Check sheet for the modelled part. Datum: model origin and axes. Units: mm. Give positions to 0.01 mm unless a question says otherwise; leave off trailing zeros. Order: outer loops, then holes, each group sorted by start corner. A loop starts at its lowest first (then second) coordinate and runs counter-clockwise, first axis right, second up.
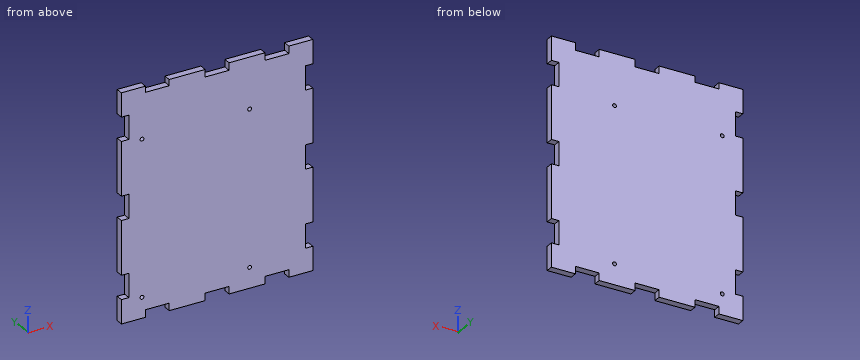
Autodesk Inventor part; units mm, degrees
ref_plane "YZ Plane" through (0, 0, 0) normal (1, 0, 0) x (0, 1, 0)
ref_plane "XZ Plane" through (0, 0, 0) normal (0, 1, 0) x (-1, 0, 0)
ref_plane "XY Plane" through (0, 0, 0) normal (0, 0, 1) x (1, 0, 0)
sketch "Fundo" plane through (0, 0, 0) normal (0, 1, 0) x (-1, 0, 0)
  line L0 (0, 0) -> (-80, 0)
  line L1 (-80, 0) -> (-80, -95)
  line L2 (-80, -95) -> (0, -95)
  line L3 (0, -95) -> (0, 0)
  dimension "d0" = 80
  dimension "d1" = 95
extrude "Extrusão1" add sketch "Fundo" along normal blind 3
sketch "Esboço3" plane through (0, 3, 0) normal (0, 1, 0) x (1, 0, 0)
  line L0 (10, -0.55) -> (20, -0.55)
  line L1 (20, -0.55) -> (20, 2.55)
  line L2 (20, 2.55) -> (10, 2.55)
  line L3 (10, 2.55) -> (10, -0.55)
  line L4 (0, 0) -> (80, 0)
  line L5 (70, 0) -> (60, 0)
  line L6 (60, 0) -> (60, 3.1)
  line L7 (60, 3.1) -> (70, 3.1)
  line L8 (70, 3.1) -> (70, 0)
  line L9 (35, 0) -> (45, 0)
  line L10 (45, 0) -> (45, 3.1)
  line L11 (45, 3.1) -> (35, 3.1)
  line L12 (35, 3.1) -> (35, 0)
  line L13 (80, 95) -> (0, 95)
  line L14 (10, 95) -> (20, 95)
  line L15 (20, 95) -> (20, 91.9)
  line L16 (20, 91.9) -> (10, 91.9)
  line L17 (10, 91.9) -> (10, 95)
  line L18 (35, 95) -> (45, 95)
  line L19 (45, 95) -> (45, 91.9)
  line L20 (45, 91.9) -> (35, 91.9)
  line L21 (35, 91.9) -> (35, 95)
  line L22 (60, 95) -> (70, 95)
  line L23 (70, 95) -> (70, 91.9)
  line L24 (70, 91.9) -> (60, 91.9)
  line L25 (60, 91.9) -> (60, 95)
  line L26 (80, 0) -> (80, 95)
  line L27 (0, 95) -> (0, 0)
  point P0 (10, 1)
  point P1 (60, 1.55)
  point P2 (20, 1)
  point P3 (35, 1.55)
  point P4 (10, 93.45)
  point P5 (70, 93.45)
  point P6 (60, 93.45)
  point P7 (45, 93.45)
  point P8 (45, 1.55)
  point P9 (35, 93.45)
  point P10 (20, 93.45)
  point P11 (20, 95)
  point P12 (45, 0)
  point P13 (60, 0)
  point P14 (70, 1.55)
  dimension "d4" = 10
  dimension "d5" = 3.1
  dimension "d7" = 10
  dimension "d8" = 3.1
  dimension "d10" = 10
  dimension "d11" = 3.1
  dimension "d18" = 10
  dimension "d19" = 3.1
  dimension "d20" = 10
  dimension "d21" = 3.1
  dimension "d22" = 10
  dimension "d23" = 3.1
  dimension "d30" = 10
  dimension "d113" = 10
  dimension "d114" = 10
  dimension "d115" = 15
  dimension "d116" = 15
  dimension "d117" = 40
  dimension "d118" = 15
  dimension "d119" = 15
  dimension "d120" = 10
extrude "Extrusão2" cut sketch "Esboço3" against normal blind 10 contours L3 L4 L1 L0 | L3 L2 L1 L4 | L12 L11 L10 L4 | L13 L15 L16 L17 | L6 L7 L8 L4 | L13 L19 L20 L21 | L13 L23 L24 L25
sketch "Esboço4" plane through (0, 3, 0) normal (0, 1, 0) x (1, 0, 0)
  line L0 (0, 95) -> (0, 0)
  line L1 (0, 10) -> (3.1, 10)
  line L2 (3.1, 10) -> (3.1, 20)
  line L3 (3.1, 20) -> (0, 20)
  line L4 (0, 20) -> (0, 10)
  line L5 (0, 85) -> (3.1, 85)
  line L6 (3.1, 85) -> (3.1, 75)
  line L7 (3.1, 75) -> (0, 75)
  line L8 (0, 75) -> (0, 85)
  line L9 (0, 42.5) -> (3.1, 42.5)
  line L10 (3.1, 42.5) -> (3.1, 52.5)
  line L11 (3.1, 52.5) -> (0, 52.5)
  line L12 (0, 52.5) -> (0, 42.5)
  line L13 (10, 95) -> (0, 95)
  line L14 (80, 0) -> (80, 95)
  line L15 (80, 10) -> (76.9, 10)
  line L16 (76.9, 10) -> (76.9, 20)
  line L17 (76.9, 20) -> (80, 20)
  line L18 (80, 20) -> (80, 10)
  line L19 (80, 42.5) -> (76.9, 42.5)
  line L20 (76.9, 42.5) -> (76.9, 52.5)
  line L21 (76.9, 52.5) -> (80, 52.5)
  line L22 (80, 52.5) -> (80, 42.5)
  line L23 (80, 75) -> (76.9, 75)
  line L24 (76.9, 75) -> (76.9, 85)
  line L25 (76.9, 85) -> (80, 85)
  line L26 (80, 85) -> (80, 75)
  line L27 (70, 0) -> (80, 0)
  line L28 (80, 95) -> (70, 95)
  point P0 (1.55, 10)
  point P1 (1.55, 85)
  point P2 (1.55, 75)
  point P3 (1.55, 52.5)
  point P4 (1.55, 20)
  point P5 (78.45, 10)
  point P6 (78.45, 85)
  point P7 (78.45, 52.5)
  point P8 (78.45, 75)
  point P9 (80, 85)
  point P10 (0, 75)
  point P11 (0, 52.5)
  point P12 (0, 20)
  point P13 (78.45, 42.5)
  point P14 (78.45, 20)
  dimension "d44" = 3.1
  dimension "d45" = 10
  dimension "d46" = 10
  dimension "d47" = 3.1
  dimension "d48" = 10
  dimension "d49" = 10
  dimension "d50" = 10
  dimension "d51" = 22.5
  dimension "d53" = 3.1
  dimension "d54" = 10
  dimension "d55" = 3.1
  dimension "d56" = 10
  dimension "d57" = 3.1
  dimension "d58" = 10
  dimension "d59" = 10
  dimension "d60" = 10
  dimension "d61" = 22.5
  dimension "d64" = 22.5
  dimension "d130" = 55
extrude "Extrusão3" cut sketch "Esboço4" against normal blind 10
sketch "Esboço6" plane through (0, 3, 0) normal (0, 1, 0) x (1, 0, 0)
  line L0 (8.6, 86.4) -> (53.6, 86.4)
  line L1 (53.6, 86.4) -> (53.6, 21.4)
  line L2 (53.6, 21.4) -> (8.6, 21.4)
  line L3 (8.6, 21.4) -> (8.6, 86.4)
  line L4 (3.1, 85) -> (3.1, 75)
  line L5 (20, 91.9) -> (10, 91.9)
  circle A0 centre (53.6, 86.4) radius 0.8
  circle A1 centre (53.6, 21.4) radius 0.8
  circle A2 centre (8.6, 21.4) radius 0.8
  circle A3 centre (8.6, 86.4) radius 0.8
  point P0 (0, 0)
  point P1 (3.1, 80)
  point P2 (15, 91.9)
  dimension "d134" = 65
  dimension "d135" = 45
  dimension "d136" = 5.5
  dimension "d137" = 5.5
  dimension "d138" = 1.6
  dimension "d139" = 1.6
  dimension "d140" = 1.6
  dimension "d141" = 1.6
extrude "Extrusão4" cut sketch "Esboço6" against normal blind 10 contours L3 A3 L0 | L0 A3 L3 | A0 L1 L0 | L0 L1 A0 | A2 L2 L3 | L3 L2 A2 | A1 L2 L1 | L1 L2 A1
properties part number "Fundo"
(1) Gauge pin test, flat ends, axial feed: pin 1 Ø1 at (y, z) = (1.5, -45) entering from -X; pin 2 Ø1.5 at (x, y) = (67, 1.5) entering from +Z. Record the tip position at first contact, or that the pin passes through.
Response values:
pin 1: stops at x = 3.1
pin 2: stops at z = -3.1
(2) Material ranges on L1, parallel to Z at x = 53.6, y = 0.9; L2, parallel to X at y = 1.75, z = -47; L3, parallel to Z at x = 53, y = 2.4, recorded low to high.
Response values:
L1: z = -95 to -87.2, -85.6 to -22.2, -20.6 to 0
L2: x = 3.1 to 76.9
L3: z = -95 to -86.93, -85.87 to -21.93, -20.87 to 0
(3) Cross-section at A-A on y = 1.9. Count the separate pieces of the cut face and the enclosed holes in it, then the cut area to 3 significant figures.
Response values:
separate pieces: 1
enclosed holes: 4
area: 7,230 mm2
(4) Cross-section at C-C on x = 11.5. Enter the section's corners in (y, z), then the cut area to 3 significant figures.
Response values:
outline: (0, -91.9) - (3, -91.9) - (3, -2.55) - (0, -2.55) - close
area: 268 mm2
(5) Cross-section at B-B on z = -83.5. Enter the section's corners in (x, y).
Response values:
outline: (3.1, 0) - (76.9, 0) - (76.9, 3) - (3.1, 3) - close
